Answer from the drawing. Dimensions are ordinates in mm from the lowest x, y and z of the part. Give positions to 0.01 mm unless a question says otherwise; leave off trailing zeros. Order: outer loops, then holes, each group sorted by start corner. A loop starts at its lowest first (then second) coordinate and runs counter-clockwise, first axis right, second up. Notation, with made-up numbers: M 27,-30 L 31,-30 A16 ccw 31,-19 Z; hole C 55.5,21.25 d11. An arc over 180 degrees is marked long. One line per item, written item: value.
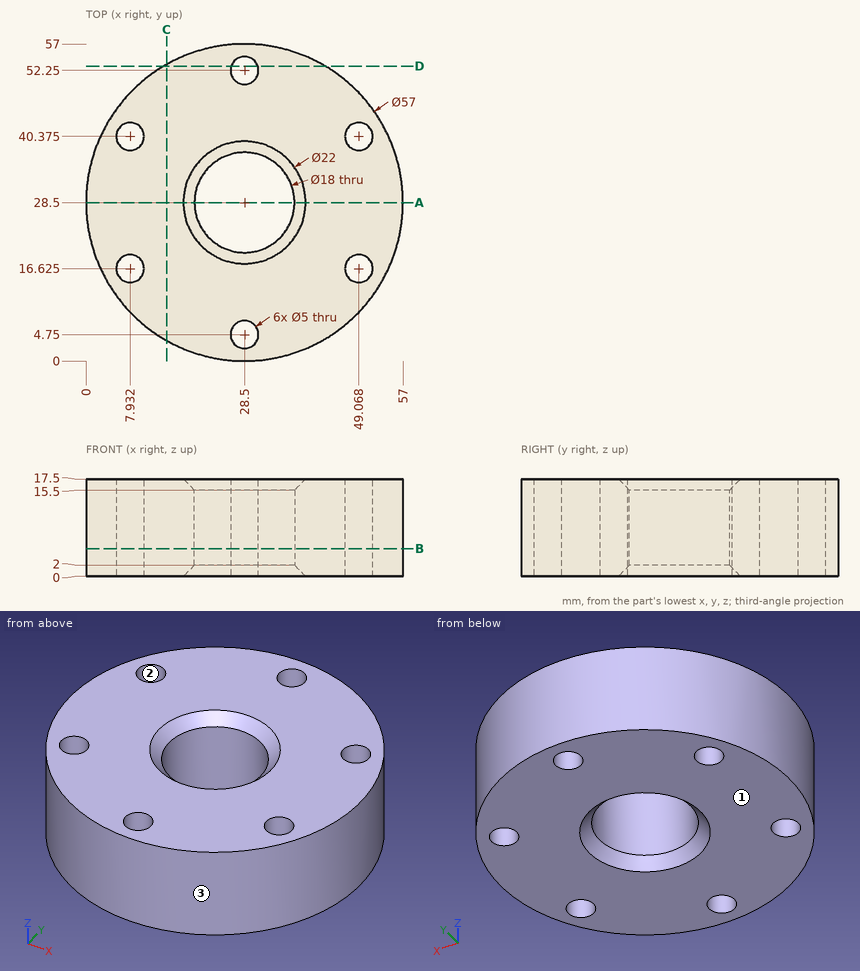
(1) Section A-A, the plane y = 28.5 is taken. Give the vertices of the cut face in (x, z), then the cut area to 4 significant figures.
Findings:
outline: M 0,0 L 17.5,0 L 19.5,2 L 19.5,15.5 L 17.5,17.5 L 0,17.5 Z; M 37.5,2 L 39.5,0 L 57,0 L 57,17.5 L 39.5,17.5 L 37.5,15.5 Z
area: 674.5 mm^2
(2) Find the intervals of material crossed by probe 1 along Y at (x, z) = (28.5, 13.25); probe 2 along X at (y, z) = (16, 11.5); probe 3 along Y at (x, z) = (47, 5), in increasing order. Write a range as from..to.
Findings:
probe 1: y = 0..2.25, 7.25..19.5, 37.5..49.75, 54.75..57
probe 2: x = 2.89..5.51, 10.35..46.65, 51.49..54.11
probe 3: y = 6.82..15.22, 18.03..38.97, 41.78..50.18
(3) Section D-D, the plane y = 53 is taken. Give the vertices of the cut face in (x, z) (3 decimals), then the cut area to 3 significant figures.
Findings:
outline: M 13.94,0 L 26.115,0 L 26.115,17.5 L 13.94,17.5 Z; M 30.885,0 L 43.06,0 L 43.06,17.5 L 30.885,17.5 Z
area: 426 mm^2
(4) Determine the mould class of the marked faces 1, 2 and 3 for opening direction X: pulls with the +X half, pulls with the -X half, needs draft (parallel to the pull), parting line crosses it, or undercut.
Findings:
face 1: needs draft
face 2: undercut
face 3: parting line crosses it
(5) Section C-C, the plane x = 14.5 is taken. Give the vertices of the cut face in (y, z).
Findings:
outline: M 3.68,0 L 53.32,0 L 53.32,17.5 L 3.68,17.5 Z
(6) Given P1, Ø6.5, axis at x = 28.5, y = 52.25, coming from the +Z side; P2, Ø8, axis at y = 45.5, z = 3.5, coming from the +X side; P3, Ø2, axis at x = 18, z = 3, coming from the -Y side; P4, Ø8, axis at y = 45.5, z = 3, coming from the -X side, each flat-ended and moving along its own axis, determine where each tip first touches the part or whether it passes through.
Findings:
P1: stops at z = 17.5
P2: stops at x = 53.86
P3: stops at y = 1.63
P4: stops at x = 3.14
(7) Section B-B, the plane z = 5 is taken. Give the vertices of the cut face in (x, y) (3 decimals), then the cut area to 3 significant figures.
Findings:
outline: C 28.5,28.5 d57; hole C 7.932,16.625 d5; hole C 7.932,40.375 d5; hole C 28.5,28.5 d18; hole C 28.5,4.75 d5; hole C 28.5,52.25 d5; hole C 49.068,16.625 d5; hole C 49.068,40.375 d5
area: 2,180 mm^2
